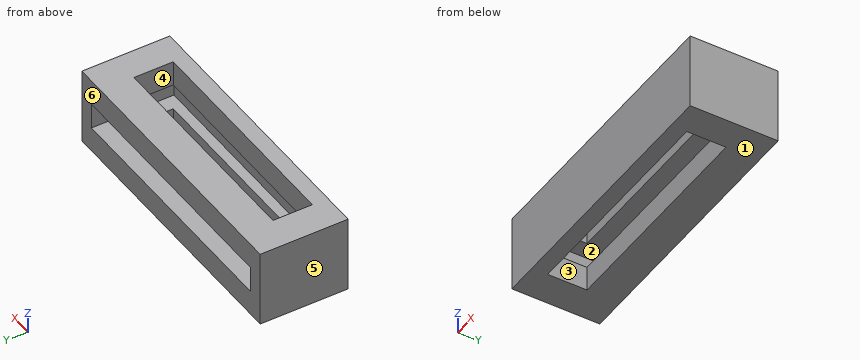
```python
from build123d import *

# Parameters (mm, degrees)
ESQUISSE1_W                  = 260
ESQUISSE1_H                  = 70
BOSS_EXTRU_1_DEPTH           = 80
ENL_V_MAT_EXTRU_1_DEPTH      = 236
ENL_V_MAT_EXTRU_1_DEPTH_BACK = 80
ESQUISSE3_W                  = 202.727222796
ESQUISSE3_H                  = 35.788236333
ESQUISSE4_W                  = 231.827281701
ESQUISSE4_H                  = 24
ENL_V_MAT_EXTRU_2_DEPTH      = 75


with BuildPart() as part:
    # Esquisse1 → Boss.-Extru.1 (new body)
    with BuildSketch(Plane(origin=(0, 0, 0), x_dir=(1, 0, 0), z_dir=(0, 1, 0))):
        with Locations((130, -35)):
            Rectangle(ESQUISSE1_W, ESQUISSE1_H)
    extrude(amount=BOSS_EXTRU_1_DEPTH)

    # Esquisse3 → Enlèv. mat.-Extru.1 (cut, two sides: drawn at the far end of the back side and taken through both)
    with BuildSketch(Plane.XY.offset(70).offset(-ENL_V_MAT_EXTRU_1_DEPTH_BACK)):
        with Locations((130.830849274, 32.105881833)):
            Rectangle(ESQUISSE3_W, ESQUISSE3_H)
    extrude(amount=ENL_V_MAT_EXTRU_1_DEPTH + ENL_V_MAT_EXTRU_1_DEPTH_BACK, mode=Mode.SUBTRACT)

    # Esquisse4 → Enlèv. mat.-Extru.2 (cut)
    with BuildSketch(Plane(origin=(0, 80, 0), x_dir=(1, 0, 0), z_dir=(0, 1, 0))):
        with Locations((130.132710296, -34.788590838)):
            Rectangle(ESQUISSE4_W, ESQUISSE4_H)
    extrude(amount=-ENL_V_MAT_EXTRU_2_DEPTH, mode=Mode.SUBTRACT)


solid = part.part
```
Build history of the part. All positions in model axes, mm. Face numbers are marked on the shaded views. A direction names the side the tool comes from. Give positions to 0.01 mm unless a question says otherwise; leave off trailing zeros. Order: outer loops, then holes, each group sorted by start corner. A loop starts at its lowest first (then second) coordinate and runs counter-clockwise, first axis right, second up. Notation, with made-up numbers: M -38,84.25 L -1,84.25 A28 ccw -1,113.25 Z; hole C 84.25,-0.5 d2. An arc over 180 degrees is marked long. Write item = value, one per line. Start each with the question number.
(1) Slice it at B-B on x = 37.5. Write the cut outline in (y, z).
(2) Which spindle directions (+Z, -Z, +X, -X, +Y, -Y) get a long thin tool onto all of the face, cutting with end or side? Do the marked faces 1, 2 and 3. Say none if no direction does.
(3) Probe L1, parallel to Z at x = 93, y = 62; L2, parallel to Y at x = 130.5, z = 19; L3, parallel to X at y = 43, z = 27. List the from-to ranges inside material, lowest first. Write a range as [from, to].
(4) Slice it at D-D on y = 64.5. Write the cut outline in (x, z), plus the area to 3 significant figures.
(5) Two-plate mould, pull along Y, no slides. Class the marked faces 4, 5 and 6: released by +Y, released by -Y, zero draft, split by the parting line, or undercut.
(6) Pin check, flat tips, straight feed: pin 1 Ø8 at (x, z) = (112.5, 47.5) entering from -Y; pin 2 Ø1 at (x, z) = (204, 46) entering from +Y. Stop position of each tip, or through.
(7) Slice it at C-C on z = 56. Write the cut outline in (x, y).
(8) Slice it at A-A on y = 20. Write the cut outline in (x, z).
Responses:
q1.outline = M 0,0 L 14.21,0 L 14.21,22.79 L 5,22.79 L 5,46.79 L 14.21,46.79 L 14.21,70 L 0,70 Z; M 50,0 L 80,0 L 80,22.79 L 50,22.79 Z; M 50,46.79 L 80,46.79 L 80,70 L 50,70 Z
q2.face_1 = -Z, +X, -X, +Y, -Y
q2.face_2 = +Y
q2.face_3 = +Z, -Z
q3.L1 = [0, 22.79], [46.79, 70]
q3.L2 = [0, 14.21], [50, 80]
q3.L3 = [0, 14.22], [246.05, 260]
q4.outline = M 0,0 L 260,0 L 260,70 L 0,70 Z; hole M 14.22,22.79 L 246.05,22.79 L 246.05,46.79 L 14.22,46.79 Z
q4.area = 12,600 mm2
q5.face_4 = undercut
q5.face_5 = zero draft
q5.face_6 = released by +Y
q6.pin_1 = 0
q6.pin_2 = 5
q7.outline = M 0,0 L 260,0 L 260,80 L 0,80 Z; hole M 29.47,14.21 L 232.19,14.21 L 232.19,50 L 29.47,50 Z
q8.outline = M 0,0 L 29.47,0 L 29.47,22.79 L 14.22,22.79 L 14.22,46.79 L 29.47,46.79 L 29.47,70 L 0,70 Z; M 232.19,0 L 260,0 L 260,70 L 232.19,70 L 232.19,46.79 L 246.05,46.79 L 246.05,22.79 L 232.19,22.79 Z
